Model file for the job. Use its own axes, mm. Face numbers are marked on the shaded views. A direction names the side the tool comes from. Round coordinates to 2 decimals unless told otherwise and drop trailing zeros. Order: outer loops, then holes, each group sorted by start corner. A loop starts at its lowest first (then second) coordinate and runs counter-clockwise, first axis right, second up. Notation, with made-up numbers: (11.5, 87.5) -> (42.5, 87.5) arc R33 cw to (42.5, 117.5) -> close; hole circle Ø10 at (77, 10). An arc over 180 degrees is marked (long way). Answer as CSV lines item,"result".
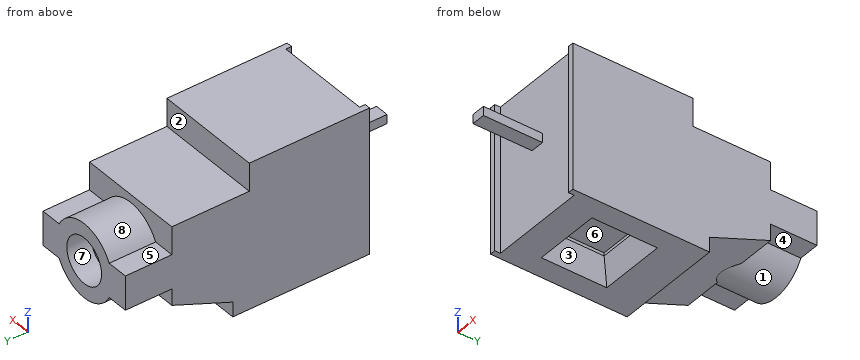
```python
from build123d import *

# Parameters (mm, degrees)
EXTRUDE_1_DEPTH      = 4.75
EXTRUDE_1_DEPTH_BACK = 4.75
EXTRUDE_START        = -4.856555
SKETCH_3_R           = 3.25
EXTRUDE_2_DEPTH      = 4.856555
SKETCH_4_R           = 2
CUT_EXTRUDE_1_DEPTH  = 2
SKETCH_7_R           = 2
SKETCH_7_R_2         = 1.8
CUT_EXTRUDE_5_DEPTH  = 0.5
SKETCH_5_W           = 4
SKETCH_5_H           = 0.464054996
CUT_EXTRUDE_2_DEPTH  = 0.5
SKETCH_8_W           = 3.834533928
SKETCH_8_H           = 3.766589268
CUT_EXTRUDE_6_DEPTH  = 2
CHAMFER_1_SIZE       = 1
CHAMFER_1_SIZE2      = 1.732050808
SKETCH_9_W           = 8.5
SKETCH_9_H           = 12.8
CUT_EXTRUDE_7_DEPTH  = 0.5
SKETCH_10_W          = 1.2
SKETCH_10_H          = 0.8
EXTRUDE_4_DEPTH      = 5.2


with BuildPart() as part:
    # 草图2 → 凸台-拉伸1 (new, two sides: drawn at the far end of the back side and taken through both)
    with BuildSketch(Plane(origin=(0, 0, 0), x_dir=(0, 0, -1), z_dir=(1, 0, 0)).offset(-EXTRUDE_1_DEPTH_BACK)):
        Polygon((6.4, 0), (-6.4, 0), (-6.4, 10.591546325), (-3.93965691, 10.591546325), (-3.93965691, 17.413010672), (-1.5, 17.413010672), (-1.5, 21.5), (1.5, 21.5), (1.5, 17.413010672), (2.939959322, 17.413010672), (5.102008026, 12.046496925), (6.4, 12.046496925), align=None)
    extrude(amount=EXTRUDE_1_DEPTH + EXTRUDE_1_DEPTH_BACK)

    # 草图3 → 凸台-拉伸2 (add)
    with BuildSketch(Plane(origin=(0, 21.5, 0), x_dir=(1, 0, 0), z_dir=(0, 1, 0)).offset(EXTRUDE_START)):
        Circle(SKETCH_3_R)
    extrude(amount=EXTRUDE_2_DEPTH)

    # 草图4 → 切除-拉伸1 (cut)
    with BuildSketch(Plane(origin=(0, 21.5, 0), x_dir=(1, 0, 0), z_dir=(0, 1, 0))):
        with Locations(Location((0, 0, 0), (0, 0, 270))):
            Circle(SKETCH_4_R)
    extrude(amount=-CUT_EXTRUDE_1_DEPTH, mode=Mode.SUBTRACT)

    # 草图7 → 切除-拉伸5 (cut)
    with BuildSketch(Plane(origin=(0, 19.5, 0), x_dir=(1, 0, 0), z_dir=(0, 1, 0))):
        with Locations(Location((0, 0, 0), (0, 0, 270))):
            Circle(SKETCH_7_R)
        with Locations(Location((0, 0, 0), (0, 0, 270))):
            Circle(SKETCH_7_R_2, mode=Mode.SUBTRACT)
    extrude(amount=-CUT_EXTRUDE_5_DEPTH, mode=Mode.SUBTRACT)

    # 草图5 → 切除-拉伸2 (cut)
    with BuildSketch(Plane(origin=(0, 19.5, 0), x_dir=(1, 0, 0), z_dir=(0, 1, 0))):
        Rectangle(SKETCH_5_W, SKETCH_5_H)
    extrude(amount=-CUT_EXTRUDE_2_DEPTH, mode=Mode.SUBTRACT)

    # 草图8 → 切除-拉伸6 (cut)
    with BuildSketch(Plane(origin=(0, 0, -6.4), x_dir=(-1, 0, 0), z_dir=(0, 0, -1))):
        with Locations((0, 5.966845297)):
            Rectangle(SKETCH_8_W, SKETCH_8_H)
    extrude(amount=-CUT_EXTRUDE_6_DEPTH, mode=Mode.SUBTRACT)

    # 倒角1
    chamfer_1_edges = [part.edges().sort_by_distance(p)[0] for p in [
        (1.917266964, 5.966845297, -6.4),
        (0, 4.083550663, -6.4),
        (-1.917266964, 5.966845297, -6.4),
        (0, 7.850139931, -6.4),
    ]]
    chamfer_1_side = [part.faces().sort_by_distance(p)[0] for p in [
        (4.596582893, 6.023248462, -6.4),
    ]]
    chamfer(chamfer_1_edges, length=CHAMFER_1_SIZE, length2=CHAMFER_1_SIZE2, reference=chamfer_1_side[0])

    # 草图9 → 切除-拉伸7 (cut)
    with BuildSketch(Plane.XZ):
        Rectangle(SKETCH_9_W, SKETCH_9_H)
    extrude(amount=-CUT_EXTRUDE_7_DEPTH, mode=Mode.SUBTRACT)

    # 草图10 → 凸台-拉伸4 (add)
    with BuildSketch(Plane.XZ.offset(-0.5)):
        with Locations((0, 0.8)):
            Rectangle(SKETCH_10_W, SKETCH_10_H)
    extrude(amount=EXTRUDE_4_DEPTH)


solid = part.part
```
Q1. Saw through at D-D (z = 2.25). Write the cut outline in (x, y).
Checks:
outline,"(-4.75, 0) -> (-4.25, 0) -> (-4.25, 0.5) -> (4.25, 0.5) -> (4.25, 0) -> (4.75, 0) -> (4.75, 17.41) -> (2.35, 17.41) -> (2.35, 21.5) -> (-2.35, 21.5) -> (-2.35, 17.41) -> (-4.75, 17.41) -> close"
Q2. Mould opens along Y. For the marked faces 1, 2 and 3 say: +Y half, -Y half, draft (parallel to the pull), parting line (faces both ways), or undercut.
Checks:
face 1,"draft"
face 2,"+Y half"
face 3,"undercut"
Q3. Flat gauge pins, fed straight in: pin 1 (1 mm diameter, centred on x = 2, y = 7.5, fed in from -Z); pin 2 (2 mm diameter, centred on x = -3.5, y = 19, fed in from +Z); pin 3 (0.5 mm diameter, centred on x = 1, z = -1, fed in from +Y). Where does each tip first touch, or does it go through?
Checks:
pin 1,"z = -5.68"
pin 2,"z = 2.08"
pin 3,"y = 19.5"
Q4. Saw through at A-A (y = 6.75). Write the cut outline in (x, z), plus the area to 3 significant figures.
Checks:
outline,"(-4.75, -6.4) -> (-2.92, -6.4) -> (-1.92, -4.67) -> (-1.92, -4.4) -> (1.92, -4.4) -> (1.92, -4.67) -> (2.92, -6.4) -> (4.75, -6.4) -> (4.75, 6.4) -> (-4.75, 6.4) -> close"
area,"112 mm²"
Q5. Wall check: L1, parallel to Z at x = 0, y = 20.65; L2, parallel to X at y = 20.65, z = 0; L3, parallel to Y at x = 2, z = -5. Give the ranges that are in metal, low to high. Write a range as [from, to].
Checks:
L1,"[-3.25, -2], [2, 3.25]"
L2,"[-4.75, -2], [2, 4.75]"
L3,"[0.5, 3.89], [8.04, 12.3]"
Q6. Tool access for the marked faces 4, 5, 6, 7 and 8: list every direction of +Z, -Z, +X, -X, +Y, -Y with a clear straight run to the whole face (end or side of a thin tool).
Checks:
face 4,"-Z, +X, +Y"
face 5,"+Z, -X, +Y"
face 6,"-Z"
face 7,"+Y"
face 8,"+Z, +Y"
Q7. Saw through at B-B (z = 4.75). Write the cut outline in (x, y).
Checks:
outline,"(-4.75, 0) -> (-4.25, 0) -> (-4.25, 0.5) -> (4.25, 0.5) -> (4.25, 0) -> (4.75, 0) -> (4.75, 10.59) -> (-4.75, 10.59) -> close"
